Design review of the part built by this model. Coordinates are the model's own, in mm. A direction names the side the tool comes from. Round coordinates to 2 decimals unless told otherwise and drop trailing zeros. Loops run counter-clockwise (first coordinate to the right, second up) from the corner with the lowest first, then second, coordinate; pieces in that order, holes last. Notation, with made-up numbers: (84, 76) -> (101, 76) arc R15 cw to (101, 99) -> close; hole circle Ø7 at (7.5, -10). An arc over 180 degrees is marked (long way). Answer as CSV lines item,"result". Start each with the question number.
```python
from build123d import *

# Parameters (mm, degrees)
F0_R     = 50.8
F0_W     = 50.8
F0_H     = 50.8
F1_DEPTH = 12.7
F2_R     = 5.08
F3_DEPTH = 57.15


with BuildPart() as f1:
    # F0 (on Top) → F1 (new body)
    with BuildSketch(Plane.XY):
        Circle(F0_R)
        Rectangle(F0_W, F0_H, mode=Mode.SUBTRACT)
    extrude(amount=F1_DEPTH)

    # F2
    f2_edges = [f1.edges().sort_by_distance(p)[0] for p in [
        (50.8, 0, 6.35),
        (-50.8, 0, 0),
        (-50.8, 0, 12.7),
    ]]
    fillet(f2_edges, radius=F2_R)

    # F3 (add): a face of the model
    f3_faces = [f1.faces().sort_by_distance(p)[0] for p in [
        (-44.4268431186, 0, 0),
    ]]
    extrude(f3_faces, amount=F3_DEPTH)


solid = f1.part
```
Q1. To check wall thickness, follow probe 1 along X at (y, z) = (-10.5, -54); probe 2 along X at (y, z) = (8, -21.5); probe 3 along Y at (x, z) = (-11.5, -46.5). State the ranges of each line that lie inside material, in increasing order. Write a range as from..to.
Q2. Machinability: for faces 1 (the flat face through (0, 25.4, -22)), 2 (the flat face through (-1, -30, 12.7)), 3 (the cylindrical face through (43.61, 13.73, -28.17)), which of the approach directions +Z, -Z, +X, -X, +Y, -Y give a long, thin tool a straight path to every point of the face, cutting with its end or side? Answer none if there is none.
Q3. Add section B-B, the plane z = -13. Give the boundary of the cut face in (x, y), and give its area (3 significant figures).
Q4. Add section A-A, the plane x = 0. Give the boundary of the cut face in (y, z).
Q5. For pin 1 Ø6 at (x, z) = (35.5, -30.5) entering from +Y; pin 2 Ø5 at (y, z) = (-28.5, -43.5) entering from +X; pin 3 Ø15 at (y, z) = (6.5, -9) entering from +X, all flat-tipped, find the tip position at first contact; note any pin that passes through.
Q6. Mouldability with a two-part tool opening along Y and no side actions: class faces 4 (the flat face through (-1, -30, -57.15)), 5 (the cylindrical face through (-11.012, -49.592, 6.332)), 6 (the flat face through (0, -25.4, -22)) as pulls with the +Y half, pulls with the -Y half, needs draft (parallel to the pull), parting line crosses it, or undercut.
Worked answers:
1,probe 1,"x = -44.5..-25.4, 25.4..44.5"
1,probe 2,"x = -45.01..-25.4, 25.4..45.01"
1,probe 3,"y = -44.25..-25.4, 25.4..44.25"
2,face 1,"+Z, -Z"
2,face 2,"+Z, +X, -X, +Y, -Y"
2,face 3,"-Z"
3,outline,"circle Ø91.44 at (0, 0); hole (-25.4, -25.4) -> (25.4, -25.4) -> (25.4, 25.4) -> (-25.4, 25.4) -> close"
3,area,"3,990 mm^2"
4,outline,"(-50.8, 5.08) arc R5.08 ccw to (-45.72, 0) -> (-45.72, -57.15) -> (-25.4, -57.15) -> (-25.4, 12.7) -> (-45.72, 12.7) arc R5.08 ccw to (-50.8, 7.62) -> close; (25.4, -57.15) -> (45.72, -57.15) -> (45.72, 0) arc R5.08 ccw to (50.8, 5.08) -> (50.8, 7.62) arc R5.08 ccw to (45.72, 12.7) -> (25.4, 12.7) -> close"
5,pin 1,"stops at y = 32.16"
5,pin 2,"stops at x = 37.61"
5,pin 3,"stops at x = 45.72"
6,face 4,"needs draft"
6,face 5,"parting line crosses it"
6,face 6,"undercut"
